Source: three-view drawing plus pictorial views. Frame: mm from the lowest corner of the part. Round coordinates to 2 decimals unless told otherwise and drop trailing zeros. Loops run counter-clockwise (first coordinate to the right, second up) from the corner with the lowest first, then second, coordinate; pieces in that order, holes last. Notation, with made-up numbers: (-12, 4) -> (14, 4) arc R22 ccw to (14, 36) -> close; hole circle Ø2 at (-29, 33). An arc over 180 degrees is marked (long way). Put each result on its own line as item: value. Start each with the question number.
1. Cut plane A-A (x = 414). State how many separate pieces and enclosed holes the cut face has, then the cut area to 3 significant figures.
2. Cut plane B-B (z = 580). Return the cut outline in (x, y).
3. Material intervals for L1, parallel to X at y = 60, z = 99.5; L2, parallel to Y at x = 594, z = 94, sorted ascending.
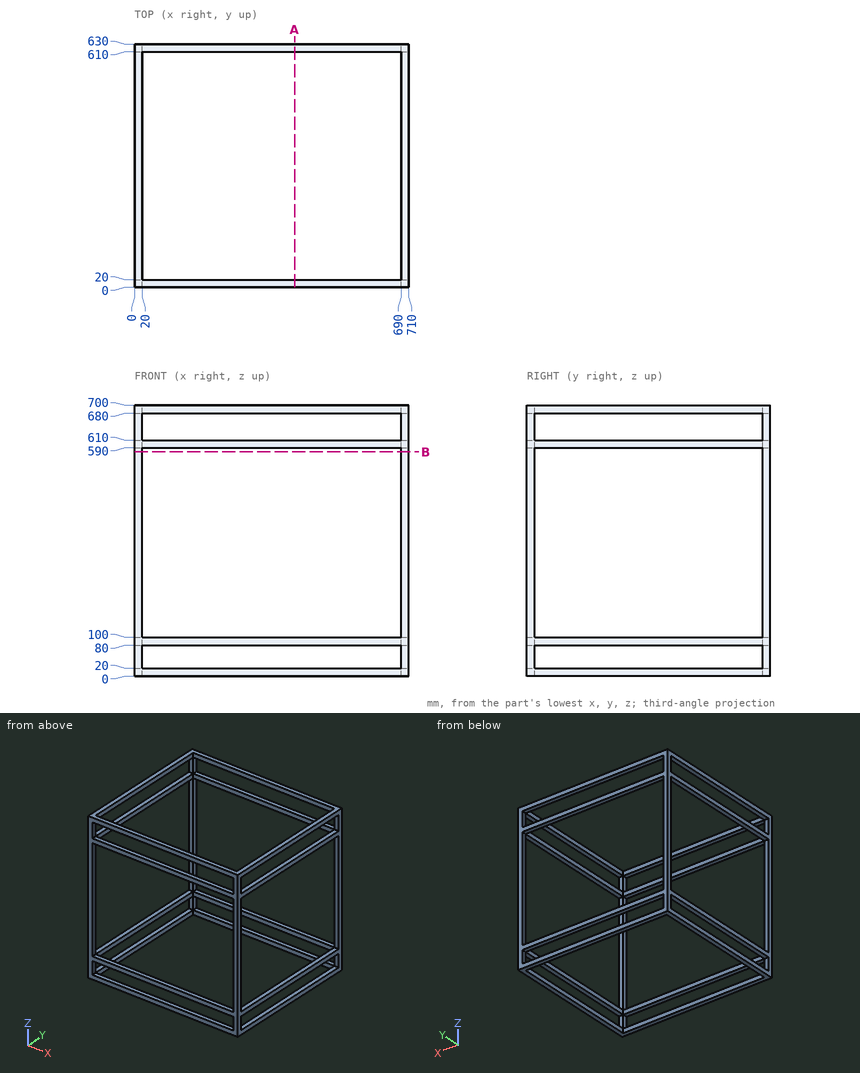
Solution:
1. separate pieces: 8
1. enclosed holes: 0
1. area: 3,200 mm^2
2. outline: (0, 0) -> (20, 0) -> (20, 20) -> (0, 20) -> close; (0, 610) -> (20, 610) -> (20, 630) -> (0, 630) -> close; (690, 0) -> (710, 0) -> (710, 20) -> (690, 20) -> close; (690, 610) -> (710, 610) -> (710, 630) -> (690, 630) -> close
3. L1: x = 0 to 20, 690 to 710
3. L2: y = 0 to 20, 610 to 630
